The listing builds one solid part. Answer for the finished solid, in the listing's coordinates (mm). A direction names the side the tool comes from. Coordinates: 2 decimals unless noted, no trailing zeros. Order: outer loops, then holes, each group sorted by start corner. A loop starts at its lowest first (then second) coordinate and runs counter-clockwise, first axis right, second up.
```python
from build123d import *

# Parameters (mm, degrees)
EXTRUDE_1_DEPTH     = 2
SKETCH_2_W          = 4
SKETCH_2_H          = 68
EXTRUDE_2_DEPTH     = 2
SKETCH_3_R          = 1
SKETCH_3_R_2        = 0.725
CUT_EXTRUDE_1_DEPTH = 5


with BuildPart() as part:
    # Model → 凸台-拉伸1 (new body)
    with BuildSketch(Plane.XY):
        Polygon((257.555719115, 185.180286748), (276.055719115, 185.180286748), (276.055719115, 187.180286748), (280.055719115, 187.180286748), (280.055719115, 185.180286748), (320.055719115, 185.180286748), (320.055719115, 187.180286748), (324.055719115, 187.180286748), (324.055719115, 185.180286748), (364.055719115, 185.180286748), (364.055719115, 187.180286748), (368.055719115, 187.180286748), (368.055719115, 185.180286748), (386.555719115, 185.180286748), (386.555719115, 173.180286748), (386.555719115, 169.180286748), (386.555719115, 137.180286748), (386.555719115, 133.180286748), (386.555719115, 121.180286748), (368.055719115, 121.180286748), (368.055719115, 119.180286748), (364.055719115, 119.180286748), (364.055719115, 121.180286748), (332.555719115, 121.180286748), (324.055719115, 121.180286748), (324.055719115, 119.180286748), (322.055719115, 119.180286748), (320.055719115, 119.180286748), (320.055719115, 121.180286748), (311.555719115, 121.180286748), (280.055719115, 121.180286748), (280.055719115, 119.180286748), (276.055719115, 119.180286748), (276.055719115, 121.180286748), (257.555719115, 121.180286748), (257.555719115, 133.180286748), (257.555719115, 137.180286748), (257.555719115, 169.180286748), (257.555719115, 173.180286748), align=None)
    extrude(amount=EXTRUDE_1_DEPTH)

    # 草图2 → 凸台-拉伸2 (add)
    with BuildSketch(Plane.XY.offset(2)):
        with Locations((366.055719115, 153.180286748)):
            Rectangle(SKETCH_2_W, SKETCH_2_H)
        with Locations((322.055719115, 153.180286748)):
            Rectangle(SKETCH_2_W, SKETCH_2_H)
        with Locations((278.055719115, 153.180286748)):
            Rectangle(SKETCH_2_W, SKETCH_2_H)
    extrude(amount=EXTRUDE_2_DEPTH)

    # 草图3 → 切除-拉伸1 (cut)
    with BuildSketch(Plane.XY.offset(2)):
        with Locations((259.055719115, 183.680286748)):
            Circle(SKETCH_3_R)
        with Locations((385.055719115, 183.680286748)):
            Circle(SKETCH_3_R)
        with Locations((385.055719115, 122.680286748)):
            Circle(SKETCH_3_R)
        with Locations((259.055719115, 122.680286748)):
            Circle(SKETCH_3_R_2)
    extrude(amount=-CUT_EXTRUDE_1_DEPTH, mode=Mode.SUBTRACT)


solid = part.part
```
(1) Find section A-A (z = 2.6). Write down the section's boundary in (x, y).
(2) For faces 3 (the face through (377, 154, 2)), 4 (the face through (344, 154, 2)), 5 (the face through (278, 154, 4)), 6 (the face through (267, 154, 2)), determine the directions among +Z, -Z, +X, -X, +Y, -Y from which every point of the face is accessible in a straight line to the end or side of a thin tool.
(3) Find section B-B (y = 127). Write down the section's boundary in (x, z).
(4) The mould has two halves that part along X. Classify faces 1 (the face through (322, 187.18, 2)), 2 (the face through (320.056, 153, 3)): released by +X, released by -X, zero draft, split by the parting line, or undercut.
(5) Each of these flat-tipped pins is pushed along its axis until it touches: pin 1 Ø1.3 at (x, y) = (259.06, 122.68) entering from -Z; pin 2 Ø4 at (x, y) = (361.5, 170.5) entering from -Z; pin 3 Ø1 at (x, z) = (268.5, 1) entering from -Y; pin 4 Ø1 at (x, z) = (265.5, 1) entering from +Y. Where does it stop, or does it pass through?
(6) Consider line 1 (X direction, y = 158, z = 2.75); line 2 (Z direction, x = 276, y = 143); line 3 (Y direction, x = 372, z = 0.2). Determine where each line is inside the solid, lowest interval first.
(7) Find section C-C (x = 339). Write down the section's boundary in (y, z), and give its area (3 significant figures).
Findings below:
1. outline: (276.06, 119.18) - (280.06, 119.18) - (280.06, 187.18) - (276.06, 187.18) - close; (320.06, 119.18) - (324.06, 119.18) - (324.06, 187.18) - (320.06, 187.18) - close; (364.06, 119.18) - (368.06, 119.18) - (368.06, 187.18) - (364.06, 187.18) - close
2. face 3: +Z, +X, +Y, -Y
2. face 4: +Z, +Y, -Y
2. face 5: +Z, +X, -X, +Y, -Y
2. face 6: +Z, -X, +Y, -Y
3. outline: (257.56, 0) - (386.56, 0) - (386.56, 2) - (368.06, 2) - (368.06, 4) - (364.06, 4) - (364.06, 2) - (324.06, 2) - (324.06, 4) - (320.06, 4) - (320.06, 2) - (280.06, 2) - (280.06, 4) - (276.06, 4) - (276.06, 2) - (257.56, 2) - close
4. face 1: zero draft
4. face 2: undercut
5. pin 1: passes through
5. pin 2: stops at z = 0
5. pin 3: stops at y = 121.18
5. pin 4: stops at y = 185.18
6. line 1: x = 276.06 to 280.06, 320.06 to 324.06, 364.06 to 368.06
6. line 2: z = 0 to 2
6. line 3: y = 121.18 to 185.18
7. outline: (121.18, 0) - (185.18, 0) - (185.18, 2) - (121.18, 2) - close
7. area: 128 mm2
